Autodesk Inventor part; units mm, degrees
ref_plane "YZ Plane" through (0, 0, 0) normal (1, 0, 0) x (0, 1, 0)
ref_plane "XZ Plane" through (0, 0, 0) normal (0, 1, 0) x (-1, 0, 0)
ref_plane "XY Plane" through (0, 0, 0) normal (0, 0, 1) x (1, 0, 0)
sketch "Sketch1" plane through (0, 0, 0) normal (0, 0, 1) x (1, 0, 0)
  line L0 (0, 0) -> (0, 50.8)
  line L1 (0, 50.8) -> (50.8, 50.8)
  line L2 (50.8, 50.8) -> (50.8, 25.4)
  line L3 (50.8, 25.4) -> (101.6, 25.4)
  line L4 (101.6, 25.4) -> (101.6, 0)
  line L5 (101.6, 0) -> (0, 0)
  line L6 (0, 50.8) -> (12.7, 50.8) construction
  line L7 (12.7, 50.8) -> (12.7, 38.1) construction
  line L8 (12.7, 38.1) -> (38.1, 38.1) construction
  line L9 (38.1, 38.1) -> (38.1, 12.7) construction
  line L10 (38.1, 12.7) -> (12.7, 12.7) construction
  line L11 (12.7, 12.7) -> (63.5, 12.7) construction
  line L12 (63.5, 12.7) -> (88.9, 12.7) construction
  circle A0 centre (12.7, 38.1) radius 2.54
  circle A1 centre (38.1, 38.1) radius 2.54
  circle A2 centre (38.1, 12.7) radius 2.54
  circle A3 centre (12.7, 12.7) radius 2.54
  circle A4 centre (63.5, 12.7) radius 2.54
  circle A5 centre (88.9, 12.7) radius 2.54
  dimension "d0" = 50.8
  dimension "d1" = 50.8
  dimension "d2" = 25.4
  dimension "d3" = 50.8
  dimension "d4" = 12.7
  dimension "d5" = 12.7
  dimension "d6" = 25.4
  dimension "d8" = 25.4
  dimension "d9" = 25.4
  dimension "d10" = 50.8
  dimension "d11" = 25.4
  dimension "d12" = 5.08
extrude "Extrusion1" add sketch "Sketch1" along normal blind 3.175
fillet "Fillet1" radius 3.175 6 edges at (50.8, 50.8, 1.5875) (50.8, 25.4, 1.5875) (0, 50.8, 1.5875) (0, 0, 1.5875) (101.6, 0, 1.5875) (101.6, 25.4, 1.5875)
properties part number "Sax Gusset" material "Aluminum 6061"
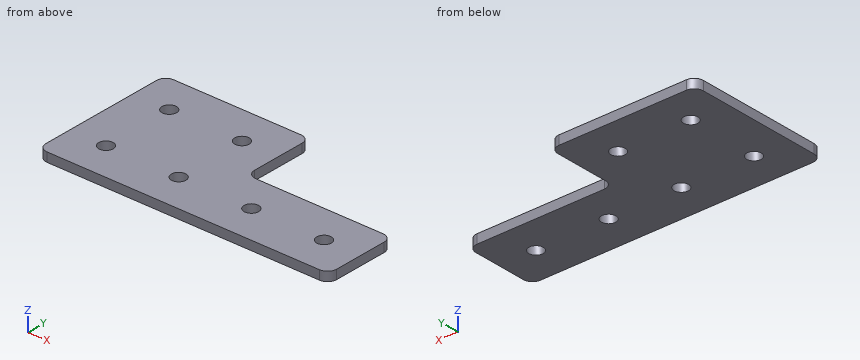
Verification items for the finished model (mm, model axes). Give positions to 0.01 mm unless a question says otherwise; leave off trailing zeros. Order: outer loops, then holes, each group sorted by start corner. A loop starts at its lowest first (then second) coordinate and runs counter-clockwise, first axis right, second up. Notation, with made-up numbers: M 82,27.25 L 127,27.25 A21 ccw 127,46.25 Z; hole C 81.25,-33 d11. An arc over 180 degrees is marked long. Answer as a JSON object with one key per item and string values. Group by question number.
1) Cross-section at A-A (x = 63.5). Enter the section's corners in (y, z) (3 decimals).
2) Cross-section at D-D (y = 38.1). Enter the section's corners in (x, z) (3 decimals).
3) Depth check by flat-ended pin: pin 1 Ø6 at (x, y) = (12.7, 38.1) entering from -Z. Enter the tip coordinate at first touch or a pass-through.
4) Cross-section at C-C (z = 2.35). Enter the section's corners in (x, y) (3 decimals), then the cut area to 3 significant figures.
5) Cross-section at B-B (y = 12.7). Enter the section's corners in (x, z) (3 decimals).
6) Scan lines: line 1 along Y through (x, z) = (12.7, 1.55); line 2 along Y through (x, z) = (89, 1); line 3 along X through (y, z) = (41.5, 1.5). Record each from-to range of solid material in increasing order. Write a range as [from, to].
Result sheet:
{
 "1": {"outline": "M 0,0 L 10.16,0 L 10.16,3.175 L 0,3.175 Z; M 15.24,0 L 25.4,0 L 25.4,3.175 L 15.24,3.175 Z"},
 "2": {"outline": "M 0,0 L 10.16,0 L 10.16,3.175 L 0,3.175 Z; M 15.24,0 L 35.56,0 L 35.56,3.175 L 15.24,3.175 Z; M 40.64,0 L 50.8,0 L 50.8,3.175 L 40.64,3.175 Z"},
 "3": {"pin 1": "stops at z = 0"},
 "4": {"outline": "M 0,3.175 A3.175 ccw 3.175,0 L 98.425,0 A3.175 ccw 101.6,3.175 L 101.6,22.225 A3.175 ccw 98.425,25.4 L 53.975,25.4 A3.175 cw 50.8,28.575 L 50.8,47.625 A3.175 ccw 47.625,50.8 L 3.175,50.8 A3.175 ccw 0,47.625 Z; hole C 12.7,12.7 d5.08; hole C 12.7,38.1 d5.08; hole C 38.1,12.7 d5.08; hole C 38.1,38.1 d5.08; hole C 63.5,12.7 d5.08; hole C 88.9,12.7 d5.08", "area": "3,740 mm2"},
 "5": {"outline": "M 0,0 L 10.16,0 L 10.16,3.175 L 0,3.175 Z; M 15.24,0 L 35.56,0 L 35.56,3.175 L 15.24,3.175 Z; M 40.64,0 L 60.96,0 L 60.96,3.175 L 40.64,3.175 Z; M 66.04,0 L 86.36,0 L 86.36,3.175 L 66.04,3.175 Z; M 91.44,0 L 101.6,0 L 101.6,3.175 L 91.44,3.175 Z"},
 "6": {"line 1": "y = [0, 10.16], [15.24, 35.56], [40.64, 50.8]", "line 2": "y = [0, 10.16], [15.24, 25.4]", "line 3": "x = [0, 50.8]"}
}
